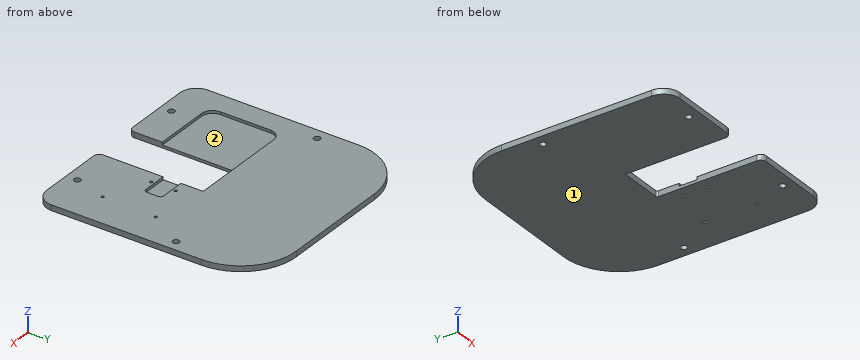
```python
from build123d import *

# Parameters (mm, degrees)
SKETCH_1_W             = 200
SKETCH_1_H             = 200
EXTRUDE_1_DEPTH        = 5
SKETCH_2_W             = 40
SKETCH_2_H             = 95
CUT_EXTRUDE_1_DEPTH    = 149.744747806
FILLET_1_R             = 50
FILLET_2_R             = 1.5
M3X0_5_1_D             = 2.5
M3X0_5_1_DEPTH         = 5
M3X0_5_1_TIP           = 0.751075774
FILLET_3_R             = 15
FILLET_4_R             = 5
HOLE_WIZARD_M5_1_D     = 5.8
HOLE_WIZARD_M5_1_DEPTH = 5
HOLE_WIZARD_M5_1_TIP   = 1.742495795
SKETCH_10_W            = 60
SKETCH_10_H            = 65
CUT_EXTRUDE_2_DEPTH    = 2.5
FILLET_5_R             = 10
SKETCH_11_W            = 25
SKETCH_11_H            = 16
CUT_EXTRUDE_3_DEPTH    = 2.5
FILLET_6_R             = 3


with BuildPart() as part:
    # ｽｹｯﾁ1 → ﾎﾞｽ - 押し出し1 (new body)
    with BuildSketch(Plane.XY):
        with Locations((0, 10)):
            Rectangle(SKETCH_1_W, SKETCH_1_H)
    extrude(amount=EXTRUDE_1_DEPTH)

    # ｽｹｯﾁ2 → ｶｯﾄ - 押し出し1 (cut, through all)
    with BuildSketch(Plane.XY.offset(5)):
        with Locations((0, -42.5)):
            Rectangle(SKETCH_2_W, SKETCH_2_H)
    extrude(amount=-CUT_EXTRUDE_1_DEPTH, mode=Mode.SUBTRACT)

    # ﾌｨﾚｯﾄ1
    fillet_1_edges = [part.edges().sort_by_distance(p)[0] for p in [
        (-100, 110, 2.5),
        (100, 110, 2.5),
    ]]
    fillet(fillet_1_edges, radius=FILLET_1_R)

    # ﾌｨﾚｯﾄ2
    fillet_2_edges = [part.edges().sort_by_distance(p)[0] for p in [
        (20, 5, 2.5),
    ]]
    fillet(fillet_2_edges, radius=FILLET_2_R)

    # M3x0.5 ねじ穴用ねじ下穴ﾄﾞﾘﾙ1
    with Locations(Plane.XY.offset(5)):
        with Locations((70, -2.5), (31, -12), (31, -34), (69, -51)):
            Hole(M3X0_5_1_D / 2, depth=M3X0_5_1_DEPTH)
            with Locations((0, 0, -(M3X0_5_1_DEPTH + M3X0_5_1_TIP / 2))):  # 118° drill point
                Cone(0, M3X0_5_1_D / 2, M3X0_5_1_TIP, mode=Mode.SUBTRACT)

    # ﾌｨﾚｯﾄ3
    fillet_3_edges = [part.edges().sort_by_distance(p)[0] for p in [
        (100, -90, 2.5),
        (-100, -90, 2.5),
    ]]
    fillet(fillet_3_edges, radius=FILLET_3_R)

    # ﾌｨﾚｯﾄ4
    fillet_4_edges = [part.edges().sort_by_distance(p)[0] for p in [
        (-20, -90, 2.5),
        (20, -90, 2.5),
    ]]
    fillet(fillet_4_edges, radius=FILLET_4_R)

    # M5 すきま穴1
    with Locations(Plane(origin=(0, 0, 0), x_dir=(-1, 0, 0), z_dir=(0, 0, -1))):
        with Locations((-60, -80), (60, -80), (-90, 30), (90, 30)):
            Hole(HOLE_WIZARD_M5_1_D / 2, depth=HOLE_WIZARD_M5_1_DEPTH)
            with Locations((0, 0, -(HOLE_WIZARD_M5_1_DEPTH + HOLE_WIZARD_M5_1_TIP / 2))):  # 118° drill point
                Cone(0, HOLE_WIZARD_M5_1_D / 2, HOLE_WIZARD_M5_1_TIP, mode=Mode.SUBTRACT)

    # ｽｹｯﾁ10 → ｶｯﾄ - 押し出し2 (cut)
    with BuildSketch(Plane.XY.offset(5)):
        with Locations((-50, -27.5)):
            Rectangle(SKETCH_10_W, SKETCH_10_H)
    extrude(amount=-CUT_EXTRUDE_2_DEPTH, mode=Mode.SUBTRACT)

    # ﾌｨﾚｯﾄ5
    fillet_5_edges = [part.edges().sort_by_distance(p)[0] for p in [
        (-80, -60, 3.75),
        (-80, 5, 3.75),
    ]]
    fillet(fillet_5_edges, radius=FILLET_5_R)

    # ｽｹｯﾁ11 → ｶｯﾄ - 押し出し3 (cut)
    with BuildSketch(Plane.XY.offset(5)):
        with Locations((32.5, -23)):
            Rectangle(SKETCH_11_W, SKETCH_11_H)
    extrude(amount=-CUT_EXTRUDE_3_DEPTH, mode=Mode.SUBTRACT)

    # ﾌｨﾚｯﾄ6
    fillet_6_edges = [part.edges().sort_by_distance(p)[0] for p in [
        (45, -15, 3.75),
        (45, -31, 3.75),
    ]]
    fillet(fillet_6_edges, radius=FILLET_6_R)


solid = part.part
```
Geometry check sheet. Reference: the model listing, model coordinates, mm. Face numbers are marked on the shaded views. Round coordinates to 2 decimals unless told otherwise and drop trailing zeros. Write each loop counter-clockwise with the first axis right and the second up, starting at its lowest first coordinate (ties: lowest second). Pieces come first, ordered by that corner, then holes. Notation, with made-up numbers: (-8.5, -29.75) - (44.5, -29.75) arc R24 ccw to (44.5, -6.75) - close; hole circle Ø6 at (5, 22). An arc over 180 degrees is marked (long way). Write each question's results on one line, items separated by ' | '.
(1) Depth check by flat-ended pin: pin 1 Ø18 at (x, y) = (-52.5, -40.5) entering from +Z; pin 2 Ø2 at (x, y) = (70, -2.5) entering from +Z; pin 3 Ø0.8 at (x, z) = (-51.5, 3.5) entering from +Y. Enter the tip coordinate at first touch or a pass-through.
Computed:
pin 1: stops at z = 2.5 | pin 2: passes through | pin 3: stops at y = 109.99
(2) Sectioned sample at A-A, the plane y = 30. Enter the section's corners in (x, z), plus the area to 3 significant figures.
Computed:
outline: (-100, 0) - (-92.9, 0) - (-92.9, 5) - (-100, 5) - close; (-87.1, 0) - (87.1, 0) - (87.1, 5) - (-87.1, 5) - close; (92.9, 0) - (100, 0) - (100, 5) - (92.9, 5) - close | area: 942 mm^2
(3) Sectioned sample at B-B, the plane x = -60. Enter the section's corners in (y, z), plus the area to 3 significant figures.
Computed:
outline: (-90, 0) - (-82.9, 0) - (-82.9, 5) - (-90, 5) - close; (-77.1, 0) - (108.99, 0) - (108.99, 5) - (5, 5) - (5, 2.5) - (-60, 2.5) - (-60, 5) - (-77.1, 5) - close | area: 803 mm^2
(4) Sectioned sample at C-C, the plane z = 1.5. Count the separate pieces of the cut face and the enclosed holes in it, plus the area to 3 significant figures.
Computed:
separate pieces: 1 | enclosed holes: 8 | area: 34,900 mm^2
(5) Thickness scan on probe 1 along X at (y, z) = (-12, 1.1); probe 2 along X at (y, z) = (-51, 1.7); probe 3 along Y at (x, z) = (-50, 4.1). Record the ranges inside material, lowest first. Write a range as from..to.
Computed:
probe 1: x = -100..-20, 20..29.75, 32.25..100 | probe 2: x = -100..-20, 20..67.75, 70.25..100 | probe 3: y = -90..-60, 5..110
(6) Sectioned sample at D-D, the plane y = -80. Enter the section's corners in (x, z), plus the area to 3 significant figures.
Computed:
outline: (-99.14, 0) - (-62.9, 0) - (-62.9, 5) - (-99.14, 5) - close; (-57.1, 0) - (-20, 0) - (-20, 5) - (-57.1, 5) - close; (20, 0) - (57.1, 0) - (57.1, 5) - (20, 5) - close; (62.9, 0) - (99.14, 0) - (99.14, 5) - (62.9, 5) - close | area: 733 mm^2
(7) Draft check along Y on the marked faces 1 and 2. Enter one of: pulls with the +Y half, pulls with the -Y half, needs draft (parallel to the pull), parting line crosses it, or undercut.
Computed:
face 1: needs draft | face 2: undercut
